Read the model definition and answer for the solid it produces. Units are mm, in the model's axes. Round coordinates to 2 decimals unless told otherwise and drop trailing zeros. Order: outer loops, then holes, each group sorted by start corner. A loop starts at its lowest first (then second) coordinate and runs counter-clockwise, first axis right, second up. Notation, with made-up numbers: (68.25, 12.5) - (122.25, 12.5) arc R15 ccw to (122.25, 25.5) - close; hole circle Ø11 at (3, 22.25). An arc over 180 degrees is marked (long way). One line per question, with ' | ' between items. Start each with the question number.
1) Flat-ended cylindrical pins translate along their axes: pin 1 (2 mm diameter, centred on x = -7, z = 9.5, fed in from -Y); pin 2 (2 mm diameter, centred on x = 8, z = 3, fed in from +Y) (3 decimals); pin 3 (4 mm diameter, centred on x = -10.5, z = 3.5, fed in from +Y). Find the tip coordinate at first contact, or state that the pin passes through.
2) The part is cut by section A-A, the plane z = 13.75. Give the vertices of the cut face in (x, y).
3) Straight lines are drawn through the part: line 1 (X direction, y = -55, z = 8.75); line 2 (X direction, y = -45, z = 12); line 3 (Y direction, x = -13, z = 8). For each, find the intervals that lie inside material, in ascending order. Write a range as from..to.
4) The part is cut by section B-B, the plane x = 1.5. Give the vertices of the cut face in (y, z), plus the area to 3 significant figures.
5) The part is cut by section C-C, the plane y = -67.5. Give the vertices of the cut face in (x, z), plus the area to 3 significant figures.
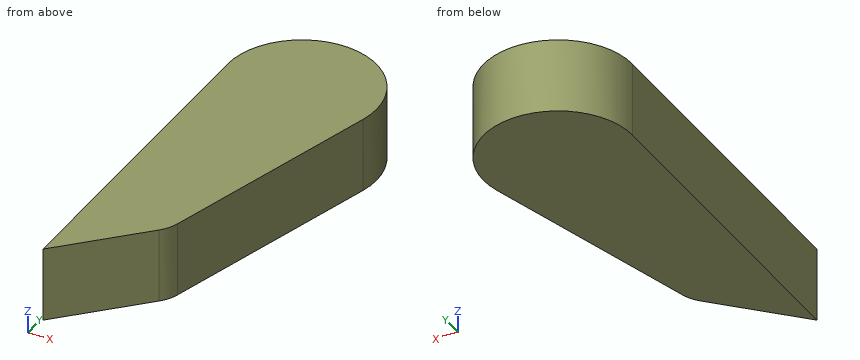
from build123d import *

# Parameters (mm, degrees)
BOSS_EXTRUDE1_DEPTH = 20


with BuildPart() as part:
    # Sketch1 → Boss-Extrude1 (new body)
    with BuildSketch(Plane.XY):
        with BuildLine():
            Line((-20, 0), (-20, -90))
            Line((-20, -90), (0, -69.709229677))
            ThreePointArc((0, -69.709229677), (1.530145443, -67.703543845), (2.509663453, -65.378750262))
            Line((2.509663453, -65.378750262), (19.263152536, -5.378750262))
            ThreePointArc((19.263152536, -5.378750262), (2.714493441, 19.814931879), (-20, 0))
        make_face()
    extrude(amount=BOSS_EXTRUDE1_DEPTH)


solid = part.part
Values:
1) pin 1: stops at y = -77.83 | pin 2: stops at y = 18.735 | pin 3: stops at y = 18.1
2) outline: (-20, -90) - (0, -69.71) arc R10 ccw to (2.51, -65.38) - (19.26, -5.38) arc R20 ccw (long way) to (-20, 0) - close
3) line 1: x = -20..5.41 | line 2: x = -20..8.2 | line 3: y = -82.9..15.2
4) outline: (-67.76, 0) - (19.94, 0) - (19.94, 20) - (-67.76, 20) - close | area: 1,750 mm^2
5) outline: (-20, 0) - (1.64, 0) - (1.64, 20) - (-20, 20) - close | area: 433 mm^2
